```python
from build123d import *

# Parameters (mm, degrees)
F0_R      = 2.5
F1_DEPTH  = 40
F2_R      = 5
F2_R_2    = 2.5
F3_DEPTH  = 3
F4_W      = 32.6441857368
F4_H      = 17.9751312453
F5_DEPTH  = 50
F6_R      = 8
F9_R      = 7
F7_R      = 5
F7_R_2    = 2.5
F10_DEPTH = 3
F11_DEPTH = 25
F12_SIZE2 = 2.5
F12_SIZE  = 2.5


with BuildPart() as f1:
    # F0 (on Front) → F1 (new body)
    with BuildSketch(Plane.XZ):
        with BuildLine():
            Line((-6.8878248776, 9.4542597632), (-14, -29.7938862443))
            Line((-14, -29.7938862443), (14, -29.7938862443))
            Line((14, -29.7938862443), (6.8878248776, 9.4542597632))
            ThreePointArc((6.8878248776, 9.4542597632), (0, 15.2061137557), (-6.8878248776, 9.4542597632))
        make_face()
        with Locations((0, 8.2061137557)):
            Circle(F0_R, mode=Mode.SUBTRACT)
        Polygon((-34, -39.7938862443), (0, -39.7938862443), (34, -39.7938862443), (34, -29.7938862443), (14, -29.7938862443), (-14, -29.7938862443), (-34, -29.7938862443), align=None)
    extrude(amount=-F1_DEPTH)

    # F2 (on face) → F3 (cut)
    with BuildSketch(Plane.XY.offset(-29.7938862443)):
        with Locations((26.0093560517, 32)):
            Circle(F2_R)
        with Locations((26.0093560517, 32)):
            Circle(F2_R_2, mode=Mode.SUBTRACT)
        with Locations((-26.0093560517, 32)):
            Circle(F2_R)
        with Locations((-26.0093560517, 32)):
            Circle(F2_R_2, mode=Mode.SUBTRACT)
        with Locations((-26.0093560517, 8)):
            Circle(F2_R)
        with Locations((-26.0093560517, 8)):
            Circle(F2_R_2, mode=Mode.SUBTRACT)
        with Locations((26.0093560517, 8)):
            Circle(F2_R)
        with Locations((26.0093560517, 8)):
            Circle(F2_R_2, mode=Mode.SUBTRACT)
    extrude(amount=-F3_DEPTH, mode=Mode.SUBTRACT)

    # F4 (on face) → F5 (cut)
    with BuildSketch(Plane.XY.offset(-29.7938862443)):
        with Locations((2.3220928684, 20)):
            Rectangle(F4_W, F4_H)
    extrude(amount=F5_DEPTH, mode=Mode.SUBTRACT)

    # F6
    f6_edges = [f1.edges().sort_by_distance(p)[0] for p in [
        (-34, 0, -34.793886),
        (34, 0, -34.793886),
        (34, 40, -34.793886),
        (-34, 40, -34.793886),
    ]]
    fillet(f6_edges, radius=F6_R)

    # F9
    f9_edges = [f1.edges().sort_by_distance(p)[0] for p in [
        (-14, 5.506217, -29.793886),
        (-14, 34.493783, -29.793886),
        (14, 5.506217, -29.793886),
        (14, 34.493783, -29.793886),
    ]]
    fillet(f9_edges, radius=F9_R)

    # F7 (on face) → F10 (join)
    with BuildSketch(Plane.XY.offset(-32.7938862443)):
        with Locations((-26.0093560517, 32)):
            Circle(F7_R)
        with Locations((-26.0093560517, 32)):
            Circle(F7_R_2, mode=Mode.SUBTRACT)
        with Locations((26.0093560517, 32)):
            Circle(F7_R)
        with Locations((26.0093560517, 32)):
            Circle(F7_R_2, mode=Mode.SUBTRACT)
        with Locations((26.0093560517, 8)):
            Circle(F7_R)
        with Locations((26.0093560517, 8)):
            Circle(F7_R_2, mode=Mode.SUBTRACT)
        with Locations((-26.0093560517, 8)):
            Circle(F7_R)
        with Locations((-26.0093560517, 8)):
            Circle(F7_R_2, mode=Mode.SUBTRACT)
    extrude(amount=F10_DEPTH)

    # F2 (on face) → F11 (cut)
    with BuildSketch(Plane.XY.offset(-29.7938862443)):
        with Locations((-26.0093560517, 32)):
            Circle(F2_R_2)
        with Locations((-26.0093560517, 8)):
            Circle(F2_R_2)
        with Locations((26.0093560517, 8)):
            Circle(F2_R_2)
        with Locations((26.0093560517, 32)):
            Circle(F2_R_2)
    extrude(amount=-F11_DEPTH, mode=Mode.SUBTRACT)

    # F12
    f12_edges = [f1.edges().sort_by_distance(p)[0] for p in [
        (-28.509356, 32, -29.793886),
        (23.509356, 32, -29.793886),
        (23.509356, 8, -29.793886),
        (-28.509356, 8, -29.793886),
    ]]
    chamfer(f12_edges, length=F12_SIZE, length2=F12_SIZE2)


solid = f1.part
```
Check sheet for the modelled part. Datum: model origin and axes. Units: mm. A direction names the side the tool comes from. Coordinates: 2 decimals unless noted, no trailing zeros. Loops run counter-clockwise (first coordinate to the right, second up) from the corner with the lowest first, then second, coordinate; pieces in that order, holes last.
1) Sectioned sample at B-B (z = -13). Record the boundary of the cut face in (x, y), and give its area (3 significant figures).
2) Sectioned sample at A-A (x = 0). Record the boundary of the cut face in (y, z), and give its area (3 significant figures).
3) Sectioned sample at D-D (y = 19). Record the boundary of the cut face in (x, z), and give its area (3 significant figures).
4) Gauge pin test, flat ends, axial feed: pin 1 (6 mm diameter, centred on x = 26.01, y = 32, fed in from +Z); pin 2 (6.5 mm diameter, centred on x = 26.01, y = 8, fed in from +Z); pin 3 (8 mm diameter, centred on x = -26.01, y = 32, fed in from +Z). Record the tip position at first contact, or that the pin passes through.
5) Sectioned sample at C-C (z = -34). Record the boundary of the cut face in (x, y), and give its area (3 significant figures).
6) Access from +Z, -Z, +X, -X, +Y, -Y to the whole of each face (thin tool, end or side, straight path). Record for faces 1 (the face through (0, 11.012, -13)), 2 (the face through (-31.719, 37.594, -34.864)).
7) Material ranges on probe 1 along Y at (x, z) = (-5, -20); probe 2 along Z at (x, y) = (0, 33.5); probe 3 along Z at (x, y) = (27, 14.5), recorded low to high.
8) Release check for a two-part mould opening along Z. For faces 3 (the face through (-9.88, 34.42, -7.06)), 4 (the face through (0, 20, -39.794)), 5 (the face through (-0.325, 34.417, 10.685)), 6 (the face through (-0.325, 5.429, 10.685)) record: released by +Z, released by -Z, zero draft, split by the parting line, or undercut.
Check sheet entries:
1. outline: (-10.96, 0) - (10.96, 0) - (10.96, 11.01) - (-10.96, 11.01) - close; (-10.96, 28.99) - (10.96, 28.99) - (10.96, 40) - (-10.96, 40) - close
1. area: 483 mm2
2. outline: (0, -39.79) - (40, -39.79) - (40, 5.71) - (28.99, 5.71) - (28.99, -29.79) - (11.01, -29.79) - (11.01, 5.71) - (0, 5.71) - close; (0, 10.71) - (11.01, 10.71) - (11.01, 15.21) - (0, 15.21) - close; (28.99, 10.71) - (40, 10.71) - (40, 15.21) - (28.99, 15.21) - close
2. area: 1,280 mm2
3. outline: (-34, -39.79) - (34, -39.79) - (34, -29.79) - (-34, -29.79) - close
3. area: 680 mm2
4. pin 1: stops at z = -31.79
4. pin 2: stops at z = -31.54
4. pin 3: stops at z = -30.79
5. outline: (-34, 8) arc R8 ccw to (-26, 0) - (26, 0) arc R8 ccw to (34, 8) - (34, 32) arc R8 ccw to (26, 40) - (-26, 40) arc R8 ccw to (-34, 32) - close; hole circle Ø5 at (-26.01, 8); hole circle Ø5 at (-26.01, 32); hole circle Ø5 at (26.01, 8); hole circle Ø5 at (26.01, 32)
5. area: 2,590 mm2
6. face 1: +Z, +X, -X
6. face 2: +Z, -Z, -X, +Y
7. probe 1: y = 0 to 11.01, 28.99 to 40
7. probe 2: z = -39.79 to 5.71, 10.71 to 15.21
7. probe 3: z = -39.79 to -29.79
8. face 3: released by +Z
8. face 4: released by -Z
8. face 5: undercut
8. face 6: undercut
